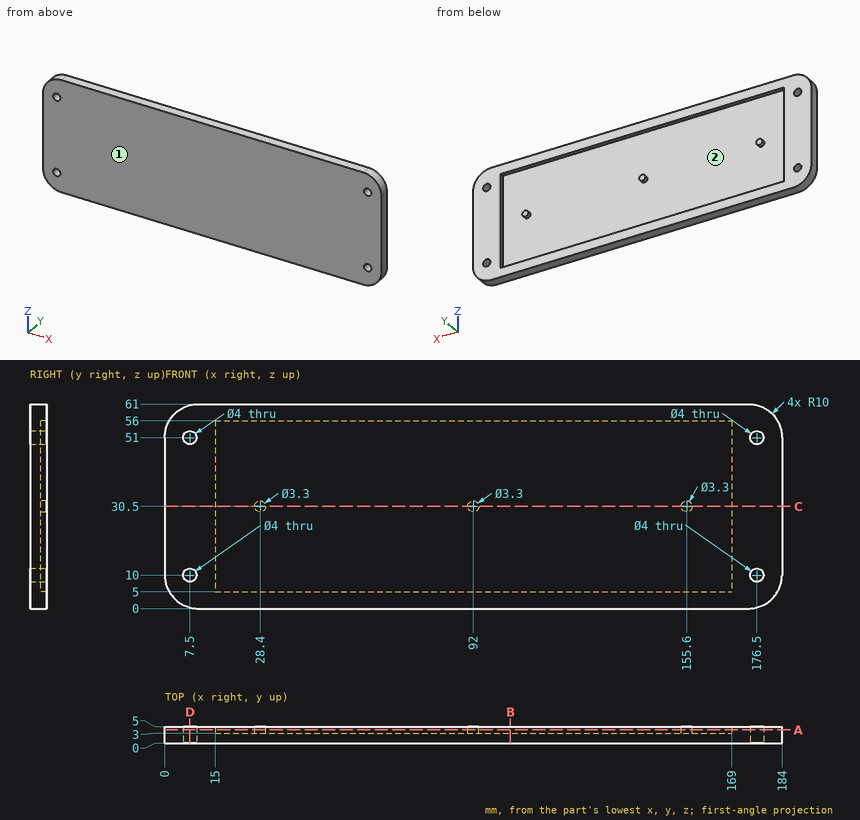
Print and shaded views of the part. All mm, measured from the part's lowest x, y and z. Coordinates: 2 decimals unless noted, no trailing zeros. Order: outer loops, then holes, each group sorted by start corner. A loop starts at its lowest first (then second) coordinate and runs counter-clockwise, first axis right, second up. Notation, with made-up numbers: M -29.75,54 L -23.75,54 A24 ccw -23.75,88 Z; hole C -10,86.25 d3. An arc over 180 degrees is marked long. One line per question, with ' | ' between items. Start each with the question number.
Q1. Two-plate mould, pull along X, no slides. Class the marked faces 1 and 2: +X half, -X half, draft (parallel to the pull), parting line (faces both ways), or undercut.
Q2. Saw through at B-B (x = 103). List the corners of the cut face in (y, z).
Q3. Saw through at C-C (z = 30.5). List the corners of the cut face in (x, y).
Q4. Saw through at A-A (y = 4). Count the separate pieces of the cut face and the enclosed holes in it, then the cut area to 3 significant figures.
Q5. Probe L1, parallel to X at y = 1.85, z = 10; L2, parallel to X at y = 3.3, z = 51; L3, parallel to Z at x = 112.5, y = 3.35. List the from-to ranges inside material, lowest first. Write a range as from..to.
Q6. Saw through at D-D (x = 7.5). List the corners of the cut face in (y, z).
Q7. Flat gauge pins, fed straight in: pin 1 Ø15.5 at (x, z) = (80.5, 42) entering from +Y; pin 2 Ø2.5 at (x, z) = (7.5, 10) entering from -Y. Where does each tip first touch, or does it go through?
Check values:
1) face 1: draft | face 2: undercut
2) outline: M 0,0 L 5,0 L 5,5 L 3,5 L 3,56 L 5,56 L 5,61 L 0,61 Z
3) outline: M 0,0 L 184,0 L 184,5 L 169,5 L 169,3 L 157.25,3 L 157.25,5 L 153.95,5 L 153.95,3 L 93.65,3 L 93.65,5 L 90.35,5 L 90.35,3 L 30.05,3 L 30.05,5 L 26.75,5 L 26.75,3 L 15,3 L 15,5 L 0,5 Z
4) separate pieces: 4 | enclosed holes: 5 | area: 3,260 mm2
5) L1: x = 0..5.5, 9.5..174.5, 178.5..184 | L2: x = 0..5.5, 9.5..15, 169..174.5, 178.5..184 | L3: z = 0..5, 56..61
6) outline: M 0,0.32 L 5,0.32 L 5,8 L 0,8 Z; M 0,12 L 5,12 L 5,49 L 0,49 Z; M 0,53 L 5,53 L 5,60.68 L 0,60.68 Z
7) pin 1: stops at y = 3 | pin 2: passes through
